Autodesk Inventor part; units mm, degrees
ref_plane "YZ Plane" through (0, 0, 0) normal (1, 0, 0) x (0, 1, 0)
ref_plane "XZ Plane" through (0, 0, 0) normal (0, 1, 0) x (-1, 0, 0)
ref_plane "XY Plane" through (0, 0, 0) normal (0, 0, 1) x (1, 0, 0)
sketch "Sketch1" plane through (0, 0, 0) normal (0, 0, 1) x (1, 0, 0)
  line L0 (27.5, 20) -> (-27.5, 20)
  line L1 (-27.5, 20) -> (-27.5, -20)
  line L2 (-27.5, -20) -> (27.5, -20)
  line L3 (27.5, -20) -> (27.5, 20)
  line L4 (27.5, 20) -> (-27.5, -20) construction
  line L5 (-27.5, 20) -> (27.5, -20) construction
  point P0 (0, 0)
  dimension "d0" = 55
  dimension "d1" = 40
extrude "Extrusion1" add sketch "Sketch1" along normal blind 3
sketch "Sketch2" plane through (0, 0, 3) normal (0, 0, 1) x (1, 0, 0)
  line L0 (27.5, 20) -> (-27.5, 20)
  line L1 (-27.5, 20) -> (-27.5, -20)
  line L2 (-27.5, -20) -> (27.5, -20)
  line L3 (27.5, -20) -> (27.5, 20)
  line L4 (-27.5, 20) -> (-24.5, 20)
  line L5 (-24.5, 20) -> (-24.5, -20)
  line L6 (-24.5, -20) -> (-27.5, -20)
  line L7 (-27.5, -20) -> (-27.5, 20)
  line L8 (27.5, 20) -> (24.5, 20)
  line L9 (24.5, 20) -> (24.5, -20)
  line L10 (24.5, -20) -> (27.5, -20)
  line L11 (27.5, -20) -> (27.5, 20)
  point P0 (0, 0)
  dimension "d4" = 3
  dimension "d5" = 3
extrude "Extrusion2" add sketch "Sketch2" along normal blind 12 contours L3 L2 L9 L0 | L5 L2 L1 L0
sketch "Sketch3" plane through (0, 0, 15) normal (0, 0, 1) x (1, 0, 0)
  line L0 (-27.5, 20) -> (-27.5, -20)
  line L1 (-27.5, -20) -> (-24.5, -20)
  line L2 (-24.5, -20) -> (-24.5, 20)
  line L3 (-24.5, 20) -> (-27.5, 20)
  line L4 (27.5, 20) -> (24.5, 20)
  line L5 (24.5, 20) -> (24.5, -20)
  line L6 (24.5, -20) -> (27.5, -20)
  line L7 (27.5, -20) -> (27.5, 20)
  line L8 (-27.5, -20) -> (27.5, -20)
  line L9 (-27.5, 20) -> (-15.5, 20)
  line L10 (-15.5, 20) -> (-15.5, -20)
  line L11 (-15.5, -20) -> (-27.5, -20)
  line L12 (-27.5, -20) -> (-27.5, 20)
  line L13 (27.5, 20) -> (15.5, 20)
  line L14 (15.5, 20) -> (15.5, -20)
  line L15 (15.5, -20) -> (27.5, -20)
  line L16 (27.5, -20) -> (27.5, 20)
  point P0 (0, 0)
  dimension "d8" = 12
  dimension "d9" = 12
extrude "Extrusion3" add sketch "Sketch3" along normal blind 3
sketch "Sketch4" plane through (0, 0, 18) normal (0, 0, 1) x (1, 0, 0)
  line L0 (-15.5, 20) -> (-27.5, 20)
  point P0 (0, 0)
  point P1 (-20, 5.5)
  point P2 (20, 5.5)
  point P3 (20, -14.5)
  point P4 (-20, -14.5)
  dimension "d12" = 40
  dimension "d13" = 20
  dimension "d14" = 14.5
  dimension "d15" = 20
hole "Hole1" at (-20, 5.5, 18) at (20, 5.5, 18) at (20, -14.5, 18) at (-20, -14.5, 18) direction (0, 0, -1) diameter 4.1 depth 8.8 tip angle 118
sketch "Sketch5" plane through (0, 0, 0) normal (0, 0, -1) x (-1, 0, 0)
  circle A0 centre (20, -14.5) radius 2.05
  circle A1 centre (20, 5.5) radius 2.05
  circle A2 centre (-20, 5.5) radius 2.05
  circle A3 centre (-20, -14.5) radius 2.05
  circle A4 centre (20, -14.5) radius 4
  circle A5 centre (-20, -14.5) radius 2.05
  circle A6 centre (-20, -14.5) radius 4
  circle A7 centre (-20, 5.5) radius 4
  circle A8 centre (20, 5.5) radius 4
  point P0 (0, 0)
  dimension "d23" = 8
  dimension "d24" = 8
  dimension "d25" = 8
  dimension "d26" = 8
extrude "Extrusion4" cut sketch "Sketch5" against normal blind 3 contours A0 | A1 | A2 | A3 | A4 | A6 | A7 | A8
sketch "Sketch6" plane through (0, 0, 0) normal (0, 0, -1) x (-1, 0, 0)
  line L0 (-27.5, 20) -> (27.5, 20)
  point P0 (0, 0)
  point P1 (5.5, 3)
  point P2 (-5.5, 3)
  point P3 (-5.5, 13)
  point P4 (5.5, 13)
  dimension "d29" = 5.5
  dimension "d30" = 11
  dimension "d31" = 10
  dimension "d56" = 7
hole "Hole2" at (-5.5, 3, 0) at (5.5, 3, 0) at (5.5, 13, 0) at (-5.5, 13, 0) direction (0, 0, 1) diameter 2.1 depth 8.8 tip angle 118
sketch "Sketch8" plane through (0, 0, 0) normal (0, 0, -1) x (-1, 0, 0)
  line L0 (24.5, 20) -> (24.5, -20)
  line L1 (27.5, 20) -> (27.5, -20)
  line L2 (-24.5, -20) -> (-24.5, 20)
  line L3 (-27.5, -20) -> (-27.5, 20)
  line L4 (27.5, -20) -> (24.5, -20)
  line L5 (24.5, -20) -> (24.5, 20)
  line L6 (24.5, 20) -> (27.5, 20)
  line L7 (27.5, 20) -> (27.5, -20)
  line L8 (27.5, -20) -> (-27.5, -20)
  line L9 (-27.5, -20) -> (-24.5, -20)
  line L10 (-24.5, -20) -> (-24.5, 20)
  line L11 (-24.5, 20) -> (-27.5, 20)
  line L12 (-27.5, 20) -> (-27.5, -20)
  point P0 (0, 0)
extrude "Extrusion5" add sketch "Sketch8" along normal blind 20
sketch "Sketch9" plane through (27.5, -20, 18) normal (1, 0, 0) x (0, 0, -1)
  point P0 (18, 20)
chamfer "Chamfer1" distance 15 angle 45 1 edges at (26, -20, -20)
chamfer "Chamfer2" distance 15 angle 45 3 edges at (26, 20, -20) (-26, -20, -20) (-26, 20, -20)
sketch "Sketch11" plane through (27.5, -20, 18) normal (1, 0, 0) x (0, 0, -1)
  line L0 (38, 25) -> (38, 15)
  point P0 (18, 20)
  point P1 (26, 20)
  dimension "d48" = 12
hole "Hole3" at (27.5, 0, -8) direction (-1, 0, 0) diameter 2.459 end through all
sketch "Sketch13" plane through (0, 0, 3) normal (0, 0, 1) x (1, 0, 0)
  line L0 (24.5, 20) -> (-24.5, 20)
  point P0 (0, 0)
  point P1 (-10, 1)
  point P2 (10, 1)
  dimension "d57" = 19
  dimension "d58" = 10
  dimension "d59" = 20
  dimension "d60" = 19
hole "Hole4" at (-10, 1, 3) at (10, 1, 3) direction (0, 0, -1) diameter 2.7 end through all
sketch "Sketch14" plane through (0, 0, 3) normal (0, 0, 1) x (1, 0, 0)
  line L0 (-8.65, -4) -> (-11.35, -4)
  line L1 (-11.35, -4) -> (-11.35, 10)
  line L2 (-11.35, 10) -> (-8.65, 10)
  line L3 (-8.65, 10) -> (-8.65, -4)
  line L4 (-8.65, -4) -> (-11.35, 10) construction
  line L5 (-11.35, -4) -> (-8.65, 10) construction
  line L6 (24.5, 20) -> (-24.5, 20)
  line L7 (11.35, 10) -> (8.65, 10)
  line L8 (8.65, 10) -> (8.65, -4)
  line L9 (8.65, -4) -> (11.35, -4)
  line L10 (11.35, -4) -> (11.35, 10)
  point P0 (0, 0)
  point P1 (-10, 3)
  point P2 (-10, 10)
  point P3 (10, 10)
  dimension "d68" = 2.7
  dimension "d69" = 10
  dimension "d70" = 7
  dimension "d71" = 10
  dimension "d72" = 2.7
  dimension "d73" = 10
  dimension "d74" = 14
  dimension "d75" = 10
extrude "Extrusion6" cut sketch "Sketch14" against normal through all
properties part number "attocube_holder" material "Koper"
Geometry: final body of the model. Coordinates: model frame, mm. A direction names the side the tool comes from. Coordinates: 2 decimals unless noted, no trailing zeros. Order: outer loops, then holes, each group sorted by start corner. A loop starts at its lowest first (then second) coordinate and runs counter-clockwise, first axis right, second up. Notation, with made-up numbers: (83.5, 4.5) - (97.5, 4.5) arc R23 cw to (97.5, 16.5) - close; hole circle Ø10 at (81.5, 51). An arc over 180 degrees is marked (long way). Return JSON: item names as keys, results as strings. Group by question number.
1. Pin query (flat end, axial travel): pin 1 (12 mm diameter, centred on x = 11.5, z = -10, fed in from +Y); pin 2 (2.5 mm diameter, centred on x = -5.5, y = 3, fed in from +Z); pin 3 (10 mm diameter, centred on x = -18, y = -3.5, fed in from -Z); pin 4 (5 mm diameter, centred on x = -20, y = 5.5, fed in from -Z). Return the tip coordinate at first contact, or that it passes through.
2. Cut plane C-C (y = 0). Count the separate pieces of the cut face and the enclosed holes in it, plus the area to 3 significant figures.
3. Set-up query: faces 4 (the face through (15.5, 0, 16)), 5 (the face through (20, 0, 15)), 6 (the face through (10, 10, 2)). Return all of +Z, -Z, +X, -X, +Y, -Y with unobstructed straight access to the full face (end or side cutting, diameter ignored); none if empty.
4. Cut plane D-D (z = 13). Output: boundary loops of the cut face in (x, y), plus the area to 3 significant figures.
5. Cut plane A-A (y = 13). Output: boundary loops of the cut face in (x, z).
6. Pull-direction query (X, two-part tool) for faces 1 (the face through (23.2, -16.9, 1.5)), 2 (the face through (27.5, 0, 3)), 3 (the face through (-22, 0, 18)); classes: pulls with the +X half, pulls with the -X half, needs draft (parallel to the pull), parting line crosses it, or undercut.
7. Cut plane B-B (x = 5.5). Output: boundary loops of the cut face in (y, z), plus the area to 3 significant figures.
8. Material intervals for line 1 along Y through (x, z) = (20, 0.7); line 2 along Y through (x, z) = (5.5, 1.55); line 3 along Z through (x, y) = (-21.5, -3), sorted ascending. Write a range as [from, to].
Resolved:
{
 "1": {"pin 1": "passes through", "pin 2": "stops at z = 3", "pin 3": "stops at z = 0", "pin 4": "stops at z = 15"},
 "2": {"separate pieces": "5", "enclosed holes": "0", "area": "398 mm²"},
 "3": {"face 4": "+Z, +Y, -Y", "face 5": "+Y, -Y", "face 6": "+Z, -Z"},
 "4": {"outline": "(-27.5, -20) - (-24.5, -20) - (-24.5, 20) - (-27.5, 20) - close; (24.5, -20) - (27.5, -20) - (27.5, 20) - (24.5, 20) - close", "area": "240 mm²"},
 "5": {"outline": "(-27.5, -12) - (-24.5, -12) - (-24.5, 0) - (-6.55, 0) - (-6.55, 3) - (-24.5, 3) - (-24.5, 15) - (-15.5, 15) - (-15.5, 18) - (-27.5, 18) - close; (-4.45, 0) - (4.45, 0) - (4.45, 3) - (-4.45, 3) - close; (6.55, 0) - (24.5, 0) - (24.5, -12) - (27.5, -12) - (27.5, 18) - (15.5, 18) - (15.5, 15) - (24.5, 15) - (24.5, 3) - (6.55, 3) - close"},
 "6": {"face 1": "undercut", "face 2": "pulls with the +X half", "face 3": "needs draft"},
 "7": {"outline": "(-20, 0) - (1.95, 0) - (1.95, 3) - (-20, 3) - close; (4.05, 0) - (11.95, 0) - (11.95, 3) - (4.05, 3) - close; (14.05, 0) - (20, 0) - (20, 3) - (14.05, 3) - close", "area": "107 mm²"},
 "8": {"line 1": "y = [-20, -18.5], [-10.5, 1.5], [9.5, 20]", "line 2": "y = [-20, 1.95], [4.05, 11.95], [14.05, 20]", "line 3": "z = [0, 3], [15, 18]"}
}
